Verification items for this drawing (mm, ordinates from the low corner). Give positions to 0.01 mm unless a question says otherwise; leave off trailing zeros. Loops run counter-clockwise (first coordinate to the right, second up) from the corner with the lowest first, then second, coordinate; pieces in that order, holes last. Notation, with made-up numbers: (58, -15) -> (85, -15) arc R16 cw to (85, -6) -> close; hole circle Ø10 at (60, 72). An arc over 180 degrees is marked (long way). Answer as a JSON object with one key per item and string values.
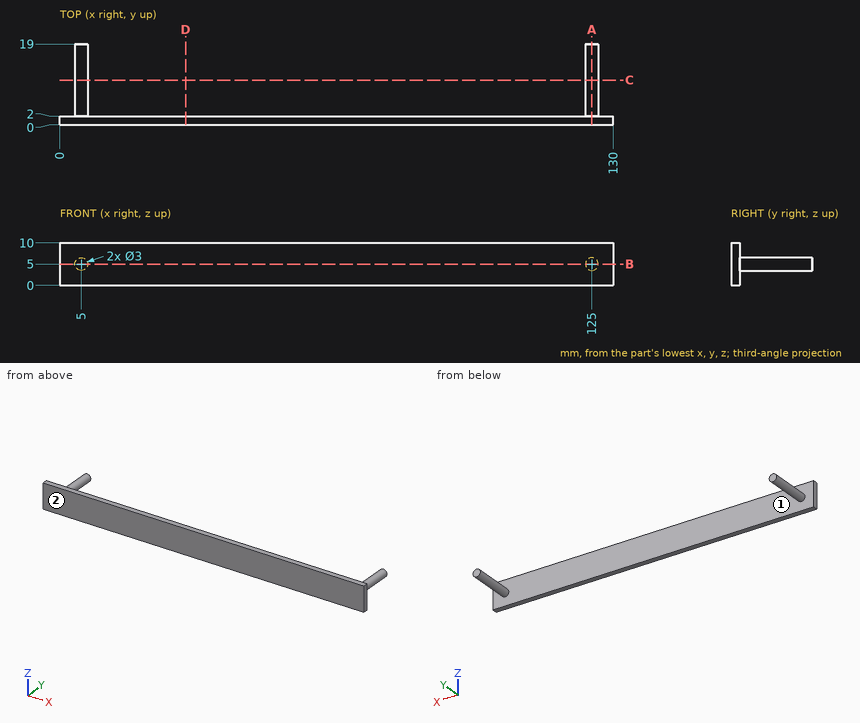
1) Section check D-D on x = 29.5. Record the cut outline in (y, z).
Geometry check:
{"outline": "(0, 0) -> (2, 0) -> (2, 10) -> (0, 10) -> close"}
2) Depth check by flat-ended pin: P1, Ø1, axis at y = 7, z = 3.5, coming from the +X side; P2, Ø6, axis at y = 10, z = 5, coming from the -X side; P3, Ø3, axis at x = 52, z = 1.5, coming from the +Y side. Enter the tip coordinate at first touch or a pass-through.
Geometry check:
{"P1": "stops at x = 126.12", "P2": "stops at x = 3.5", "P3": "stops at y = 2"}
3) Draft check along X on the marked faces 1 and 2. Enter one of: pulls with the +X half, pulls with the -X half, needs draft (parallel to the pull), parting line crosses it, or undercut.
Geometry check:
{"face 1": "undercut", "face 2": "needs draft"}
4) Material ranges on line 1 along X through (y, z) = (18.25, 5); line 2 along Y through (x, z) = (109.5, 6); line 3 along X through (y, z) = (17.75, 3.75), recorded low to high. Write a range as from..to.
Geometry check:
{"line 1": "x = 3.5..6.5, 123.5..126.5", "line 2": "y = 0..2", "line 3": "x = 4.17..5.83, 124.17..125.83"}
5) Section check A-A on x = 125. Record the cut outline in (y, z), plus the area to 3 significant figures.
Geometry check:
{"outline": "(0, 0) -> (2, 0) -> (2, 3.5) -> (19, 3.5) -> (19, 6.5) -> (2, 6.5) -> (2, 10) -> (0, 10) -> close", "area": "71.0 mm2"}
6) Section check B-B on z = 5. Record the cut outline in (x, y), plus the area to 3 significant figures.
Geometry check:
{"outline": "(0, 0) -> (130, 0) -> (130, 2) -> (126.5, 2) -> (126.5, 19) -> (123.5, 19) -> (123.5, 2) -> (6.5, 2) -> (6.5, 19) -> (3.5, 19) -> (3.5, 2) -> (0, 2) -> close", "area": "362 mm2"}
7) Section check C-C on y = 10.5. Record the cut outline in (x, z), plus the area to 3 significant figures.
Geometry check:
{"outline": "circle Ø3 at (5, 5); circle Ø3 at (125, 5)", "area": "14.1 mm2"}
